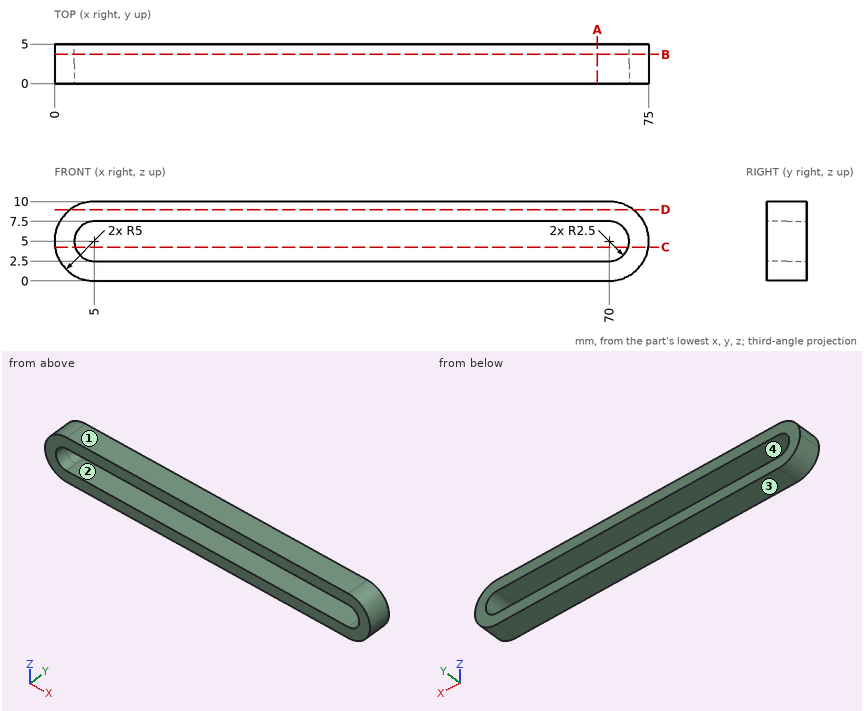
Geometry check sheet. Reference: drawing and pictorial views, mm from the part's lowest x, y, z. A direction names the side the tool comes from. Coordinates: 2 decimals unless noted, no trailing zeros. Write each loop counter-clockwise with the first axis right and the second up, starting at its lowest first coordinate (ties: lowest second). Pieces come first, ordered by that corner, then holes. Notation, with made-up numbers: M -26.75,27.5 L -11.75,27.5 A11 cw -11.75,47.5 Z; hole C 7,78 d5. An arc over 180 degrees is marked long. Use one line per item in the form item = value.
Item 1: Sectioned sample at C-C, the plane z = 4.25. Record the cut outline in (x, y).
Answer below:
outline = M 0.06,0 L 2.62,0 L 2.62,5 L 0.06,5 Z; M 72.38,0 L 74.94,0 L 74.94,5 L 72.38,5 Z
Item 2: Release check for a two-part mould opening along X. For the marked faces 1 and 2 record: pulls with the +X half, pulls with the -X half, needs draft (parallel to the pull), parting line crosses it, or undercut.
Answer below:
face_1 = needs draft
face_2 = undercut
Item 3: Sectioned sample at D-D, the plane z = 9. Record the cut outline in (x, y), and give its area (3 significant figures).
Answer below:
outline = M 2,0 L 73,0 L 73,5 L 2,5 Z
area = 355 mm^2
Item 4: Material ranges on L1, parallel to Z at x = 55, y = 1.35; L2, parallel to X at y = 0.65, z = 5.25; L3, parallel to X at y = 3.35, z = 3, recorded low to high. Write a range as from..to.
Answer below:
L1 = 0..2.5, 7.5..10
L2 = 0.01..2.51, 72.49..74.99
L3 = 0.42..3.5, 71.5..74.58
Item 5: Set-up check for the marked faces 3 and 4: record each of +Z, -Z, +X, -X, +Y, -Y from which the full face is reachable in a straight line by a thin tool's end or side.
Answer below:
face_3 = -Z, +X, -X, +Y, -Y
face_4 = +Y, -Y
Item 6: Sectioned sample at B-B, the plane y = 3.7. Record the cut outline in (x, z).
Answer below:
outline = M 5,0 L 70,0 A5 ccw 70,10 L 5,10 A5 ccw Z; hole M 5,2.5 L 70,2.5 A2.5 ccw 70,7.5 L 5,7.5 A2.5 ccw Z
Item 7: Sectioned sample at A-A, the plane x = 68.5. Record the cut outline in (y, z).
Answer below:
outline = M 0,0 L 5,0 L 5,2.5 L 0,2.5 Z; M 0,7.5 L 5,7.5 L 5,10 L 0,10 Z
Item 8: Gauge pin test, flat end, axial feed: pin 1 Ø3 at (y, z) = (3.5, 8.5) entering from +X. Record the tip position at first contact, or that the pin passes through.
Answer below:
pin_1 = 74.58
